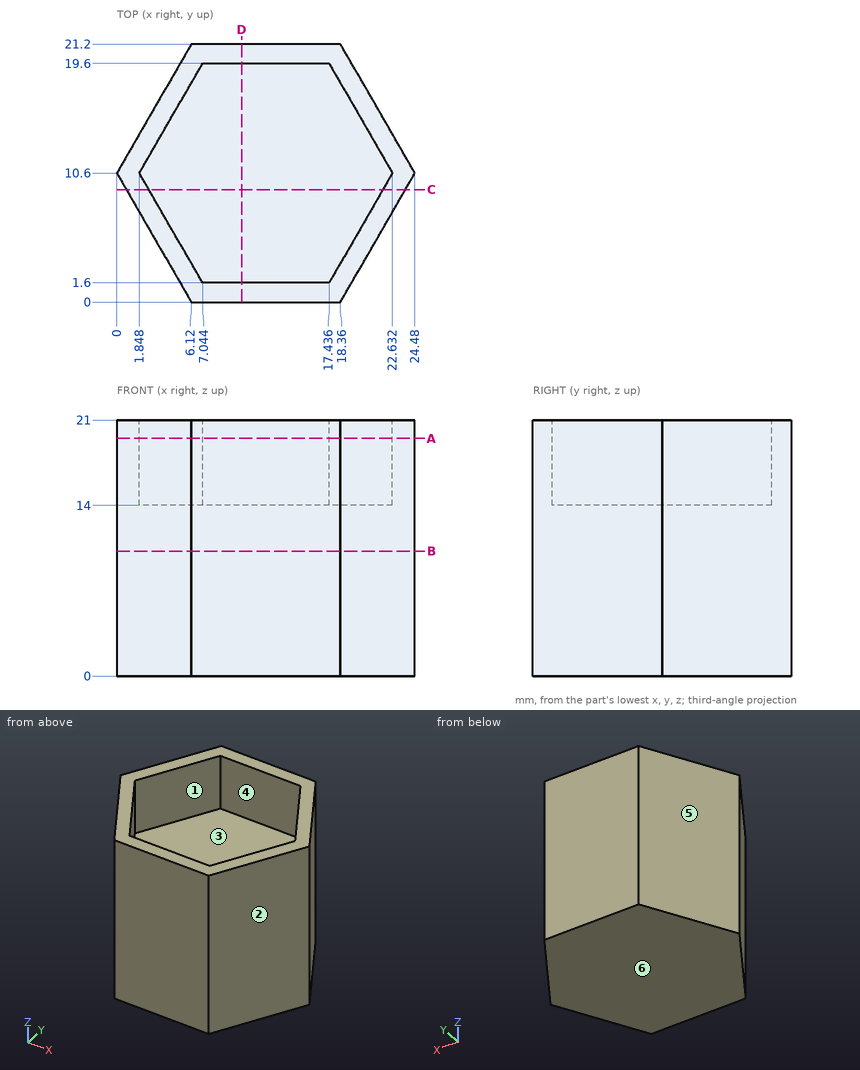
Study the drawing (mm; zero at the part's minimum x, y, z) and answer. A direction names the side the tool comes from. Give positions to 0.01 mm unless a question says otherwise; leave off trailing zeros. Loops run counter-clockwise (first coordinate to the right, second up) from the corner with the lowest first, then second, coordinate; pieces in that order, holes last. Notation, with made-up numbers: (45, 71) -> (56, 71) arc R21 cw to (56, 86) -> close; hole circle Ø9 at (49.5, -25). An arc over 180 degrees is marked (long way). Write item = value, one per line. Start each with the question number.
(1) Find the intervals of material crossed by probe 1 along Y at (x, z) = (14.25, 15.5); probe 2 along Z at (x, y) = (16.25, 3.5); probe 3 along X at (y, z) = (18.25, 14.25) (1 decimal), in increasing order. Write a range as from..to.
(2) Find section B-B on z = 10.25. Give the vertices of the cut face in (x, y), and give its area (3 significant figures).
(3) Find section A-A on z = 19.5. Give the vertices of the cut face in (x, y).
(4) Find section D-D on x = 10.25. Give the vertices of the cut face in (y, z), and give its area (3 significant figures).
(5) Find section C-C on y = 9.25. Give the vertices of the cut face in (x, z).
(6) Which of the six approach directions +Z, -Z, +X, -X, +Y, -Y give full straight-line access (tool end or side, diameter ignored) to the marked faces 1 and 2?
(7) Given pin 1 Ø1 at (x, z) = (5, 13) entering from +Y (1 decimal); pin 2 Ø1.5 at (x, z) = (5, 2.5) entering from +Y; pin 3 Ø4 at (y, z) = (15, 15.5) entering from +X (1 decimal); pin 4 Ø3 at (x, y) = (3.5, 11.5) entering from +Z, each flat-ended and moving along its own axis, determine where each tip first touches the part or whether it passes through.
(8) The mould has two halves that part along X. Classify the marked faces 3, 4, 5 and 6: +X half, -X half, draft (parallel to the pull), parting line (faces both ways), or undercut.
From the geometry:
q1.probe_1 = 0..1.6, 19.6..21.2
q1.probe_2 = 0..14
q1.probe_3 = 4.4..6.3, 18.2..20.1
q2.outline = (0, 10.6) -> (6.12, 0) -> (18.36, 0) -> (24.48, 10.6) -> (18.36, 21.2) -> (6.12, 21.2) -> close
q2.area = 389 mm^2
q3.outline = (0, 10.6) -> (6.12, 0) -> (18.36, 0) -> (24.48, 10.6) -> (18.36, 21.2) -> (6.12, 21.2) -> close; hole (1.85, 10.6) -> (7.04, 1.6) -> (17.44, 1.6) -> (22.63, 10.6) -> (17.44, 19.6) -> (7.04, 19.6) -> close
q4.outline = (0, 0) -> (21.2, 0) -> (21.2, 21) -> (19.6, 21) -> (19.6, 14) -> (1.6, 14) -> (1.6, 21) -> (0, 21) -> close
q4.area = 319 mm^2
q5.outline = (0.78, 0) -> (23.7, 0) -> (23.7, 21) -> (21.85, 21) -> (21.85, 14) -> (2.63, 14) -> (2.63, 21) -> (0.78, 21) -> close
q6.face_1 = +Z
q6.face_2 = +Z, -Z, +X, -Y
q7.pin_1 = 20.1
q7.pin_2 = 20.56
q7.pin_3 = 23.1
q7.pin_4 = 21
q8.face_3 = undercut
q8.face_4 = undercut
q8.face_5 = -X half
q8.face_6 = draft
